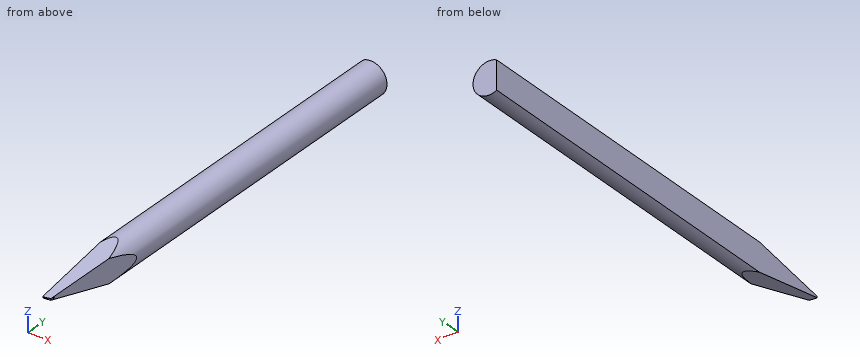
```python
from build123d import *

# Parameters (mm, degrees)
TD_SKETCH_R                             = 0.79248
TL_FEATURE_DEPTH                        = 21.0312
TDF_STD_SKETCH_W                        = 2.09296
TDF_STD_SKETCH_H                        = 2.09296
TDF_STD_FEATURE_DEPTH                   = 22.061040395
ISA_20_STD_FEATURE_DEPTH                = 22.061040395
ISA_20_STD_FEATURE_DEPTH_BACK           = 22.061040395
F_10BA_STD_FEATURE_DEPTH                = 22.061040395
F_10BA_STD_FEATURE_DEPTH_BACK           = 22.061040395
FRO_STD_FEATURE_DEPTH                   = 22.061040395
FRO_STD_FEATURE_DEPTH_BACK              = 22.061040395
C_STD_FEATURE_DEPTH                     = 22.061040395
C_STD_FEATURE_DEPTH_BACK                = 22.061040395
ERW_STD_FEATURE_DEPTH                   = 0.01905
H_STD_FEATURE_REACH                     = 22.896
H_STD_SKETCH_R                          = 0.01905
H_STD_SKETCH_3_R                        = 0.01905
FUNNEL_FINAL_DIAMETRE_STD_FEATURE_DEPTH = 2.499995
FUNNEL_FINAL_DIAMETRE_STD_FEATURE_DRAFT = -22.5
ROUND_BR_STD_FEATURE_START              = -1
ROUND_BR_STD_FEATURE_DEPTH              = 1.009339363


with BuildPart() as part:
    # TD_sketch → TL_feature (new body)
    with BuildSketch(Plane(origin=(0, 0, 0), x_dir=(1, 0, 0), z_dir=(0, 1, 0))):
        with Locations(Location((0, 0, 0), (0, 0, 270))):
            Circle(TD_SKETCH_R)
    extrude(amount=TL_FEATURE_DEPTH)

    # TDF_STD_sketch → TDF_STD_feature (cut, through all)
    with BuildSketch(Plane(origin=(0, 0, 0), x_dir=(1, 0, 0), z_dir=(0, 1, 0))):
        with Locations((-1.4224, 0)):
            Rectangle(TDF_STD_SKETCH_W, TDF_STD_SKETCH_H)
    extrude(amount=TDF_STD_FEATURE_DEPTH, mode=Mode.SUBTRACT)

    # ISA_20_STD_sketch → ISA_20_STD_feature (cut, two sides: drawn at the far end of the back side and taken through both)
    with BuildSketch(Plane(origin=(0, 0, 0), x_dir=(0, 0, -1), z_dir=(1, 0, 0)).offset(-ISA_20_STD_FEATURE_DEPTH_BACK)):
        Polygon((-12.946999885, 73.253224398), (-3.738847997, 21.0312), (-0.03048, 0), (0.03048, 0), (3.738847997, 21.0312), (12.946999885, 73.253224398), (12.946999885, -32.802042202), (-12.946999885, -32.802042202), align=None)
    extrude(amount=ISA_20_STD_FEATURE_DEPTH + ISA_20_STD_FEATURE_DEPTH_BACK, mode=Mode.SUBTRACT)

    # 10BA_STD_sketch → 10BA_STD_feature (cut, two sides: drawn at the far end of the back side and taken through both)
    with BuildSketch(Plane.XY.offset(-F_10BA_STD_FEATURE_DEPTH_BACK)):
        Polygon((-53.216424634, 0), (-0.37592, 0), (-0.29972, 0), (-0.011354365, 0.050846642), (3.688047997, 21.0312), (12.863705333, 73.068938636), (91.245889802, 2.18375769), (25.165759835, -70.885180946), align=None)
    extrude(amount=F_10BA_STD_FEATURE_DEPTH + F_10BA_STD_FEATURE_DEPTH_BACK, mode=Mode.SUBTRACT)

    # FRO_STD_sketch → FRO_STD_feature (cut, two sides: drawn at the far end of the back side and taken through both)
    with BuildSketch(Plane.XY.offset(-FRO_STD_FEATURE_DEPTH_BACK)):
        with BuildLine():
            Line((-0.37592, 52.152138388), (-0.37592, 0.02794))
            ThreePointArc((-0.37592, 0.02794), (-0.367736563, 0.008183437), (-0.34798, 0))
            Line((-0.34798, 0), (51.776218388, 0))
            Line((51.776218388, 0), (-21.9385299, -73.714748288))
            Line((-21.9385299, -73.714748288), (-74.090668288, -21.5626099))
            Line((-74.090668288, -21.5626099), (-0.37592, 52.152138388))
        make_face()
    extrude(amount=FRO_STD_FEATURE_DEPTH + FRO_STD_FEATURE_DEPTH_BACK, mode=Mode.SUBTRACT)

    # C_STD_sketch → C_STD_feature (cut, two sides: drawn at the far end of the back side and taken through both)
    with BuildSketch(Plane(origin=(0, 0, 0), x_dir=(0, 0, -1), z_dir=(1, 0, 0)).offset(-C_STD_FEATURE_DEPTH_BACK)):
        with BuildLine():
            Line((-50.530423385, -12.791040855), (-0.030559272, 0))
            ThreePointArc((-0.030559272, 0), (0, 0.00381), (0.030559272, 0))
            Line((0.030559272, 0), (50.530423385, -12.791040855))
            Line((50.530423385, -12.791040855), (50.530423385, -116.980234183))
            Line((50.530423385, -116.980234183), (-50.530423385, -116.980234183))
            Line((-50.530423385, -116.980234183), (-50.530423385, -12.791040855))
        make_face()
    extrude(amount=C_STD_FEATURE_DEPTH + C_STD_FEATURE_DEPTH_BACK, mode=Mode.SUBTRACT)


with BuildPart() as body_2:
    # ERW_STD_sketch → ERW_STD_feature (new, symmetric)
    with BuildSketch(Plane.XY):
        Polygon((-0.1397, 0.09144), (-0.1397, 0), (-0.32512, 0), (-0.272327091, 0.09144), align=None)
    extrude(amount=ERW_STD_FEATURE_DEPTH, both=True)

    # H_STD_sketch → H_STD_feature (add, up to next)
    with BuildSketch(Plane(origin=(-0.010897713, 0.165804035, 0), x_dir=(0, 0, -1), z_dir=(0.8660254037844415, 0.4999999999999953, 0)), mode=Mode.PRIVATE) as h_std_feature_sk1:
        with Locations(Location((0, 0, 0), (0, 0, 90))):
            Circle(H_STD_SKETCH_R)
    h_std_feature_tool1 = extrude(h_std_feature_sk1.sketch, amount=-H_STD_FEATURE_REACH, mode=Mode.PRIVATE) - body_2.part
    add(h_std_feature_tool1.solids().sort_by_distance((-0.010898, 0.165804, 0))[0])


with BuildPart() as funnel_final_diametre_std_feature_tool:
    # H_STD_sketch<3> → funnel_final_diametre_STD_feature (with draft: the straight prism first)
    with BuildSketch(Plane(origin=(-0.010897713, 0.165804035, 0), x_dir=(0, 0, -1), z_dir=(0.8660254037844415, 0.4999999999999953, 0))):
        with Locations(Location((0, 0, 0), (0, 0, 90))):
            Circle(H_STD_SKETCH_3_R)
    extrude(amount=FUNNEL_FINAL_DIAMETRE_STD_FEATURE_DEPTH)
    # funnel_final_diametre_STD_feature: the draft: its side faces are tilted about the plane it starts from
    funnel_final_diametre_std_feature_sides = [funnel_final_diametre_std_feature_tool.faces().sort_by_distance(p)[0] for p in [
        (1.081156877, 0.774305001, 0),
    ]]
    draft(funnel_final_diametre_std_feature_sides, Plane(origin=(-0.010897713, 0.165804035, 0), x_dir=(0, 0, -1), z_dir=(0.8660254037844415, 0.4999999999999953, 0)), FUNNEL_FINAL_DIAMETRE_STD_FEATURE_DRAFT)


with BuildPart() as body_2_1:
    add(body_2.part)

    # funnel_final_diametre_STD_feature: add funnel_final_diametre_std_feature_tool
    add(funnel_final_diametre_std_feature_tool.part)

    # ROUND_BR_STD_feature: read off the stored shape, not the designer's step
    # ROUND_BR_STD_feature outline → ROUND_BR_STD_feature (cut)
    with BuildSketch(Plane(origin=(0, 0, 0), x_dir=(0.8660254037844362, -0.5000000000000042, 0), z_dir=(0.5000000000000042, 0.8660254037844363, 0)).offset(ROUND_BR_STD_FEATURE_START)):
        with BuildLine():
            Line((-0.281562179, -0.01905), (-0.262512179, -0.01905))
            ThreePointArc((-0.262512179, -0.01905), (-0.275982563, -0.013470384), (-0.281562179, 0))
            Line((-0.281562179, 0), (-0.281562179, -0.01905))
        make_face()
        with BuildLine():
            Line((-0.281562179, 0.01905), (-0.281562179, 0))
            ThreePointArc((-0.281562179, 0), (-0.275982563, 0.013470384), (-0.262512179, 0.01905))
            Line((-0.262512179, 0.01905), (-0.281562179, 0.01905))
        make_face()
    extrude(amount=ROUND_BR_STD_FEATURE_DEPTH, mode=Mode.SUBTRACT)


with BuildPart() as part_1:
    add(part.part)

    # COMBINE_STD_feature: cut body 2
    add(body_2_1.part, mode=Mode.SUBTRACT)


solid = part_1.part
```
Check sheet for the modelled part. Datum: model origin and axes. Units: mm. Give positions to 0.01 mm unless a question says otherwise; leave off trailing zeros. Write each loop counter-clockwise with the first axis right and the second up, starting at its lowest first coordinate (ties: lowest second). Pieces come first, ordered by that corner, then holes. Notation, with made-up numbers: (-22.75, -17) -> (-6.75, -17) arc R22 cw to (-6.75, -1) -> close; hole circle Ø7 at (-38, 76.5). An arc over 180 degrees is marked (long way). Use CSV: the item, a comma, the result in double quotes. Start each with the question number.
Q1. Cross-section at C-C on z = -0.4. Enter the section's corners in (x, y).
Q2. Cross-section at A-A on y = 14.5. Enter the section's corners in (x, z), and give its area (3 significant figures).
Q3. Scan lines: line 1 along Z through (x, y) = (0.7, 13.5); line 2 along Z through (x, y) = (0.25, 2.5); line 3 along X through (y, z) = (6, 0.5). Record each from-to range of solid material in increasing order.
Q4. Cross-section at B-B on x = 0.35. Enter the section's corners in (y, z).
Working result:
1,outline,"(-0.38, 2.1) -> (0.35, 2.1) -> (0.68, 4) -> (0.68, 21.03) -> (-0.38, 21.03) -> close"
2,outline,"(-0.38, -0.7) arc R0.79 ccw (long way) to (-0.38, 0.7) -> close"
2,area,"1.56 mm^2"
3,line 1,"z = -0.37 to 0.37"
3,line 2,"z = -0.47 to 0.47"
3,line 3,"x = -0.38 to 0.61"
4,outline,"(2.1, -0.4) -> (3.86, -0.71) -> (21.03, -0.71) -> (21.03, 0.71) -> (3.86, 0.71) -> (2.1, 0.4) -> close"
